Can you work these out from the model? Positions are in its coordinate system, mm. A direction names the side the tool comes from. Coordinates: 2 decimals unless noted, no trailing zeros. Loops run counter-clockwise (first coordinate to the right, second up) from the corner with the lowest first, then second, coordinate; pieces in that order, holes last. Notation, with made-up numbers: M 72.5,-25.5 L 85.5,-25.5 A15 cw 85.5,-1.5 Z; hole C 38.5,-36.75 d7. An arc over 180 degrees is marked long. Answer as a JSON object with one key per item and string values. Group by question number.
Item 1: Suppose I cut it at A-A (y = 10.5). Write out the boundary of the cut face in (x, z).
Item 2: Suppose I cut it at D-D (x = 293). Write out the boundary of the cut face in (y, z).
Item 3: We'd pull the mould along X, two halves only. Please class faces 5 (the flat face through (330.2, 2, 452)), 6 (the flat face through (0, -75, 526)), 7 (the flat face through (153, 25.4, 526)), 8 (the flat face through (279, -77, 50.8)): +X half, -X half, draft (parallel to the pull), parting line (faces both ways), or undercut.
Item 4: Suppose I cut it at B-B (z = 438). Write out the boundary of the cut face in (x, y), then the cut area to 3 significant figures.
Item 5: If I drill on line 1 (Z direction, x = 442.5, y = -31.5); line 2 (Y direction, x = 26, z = 861); line 3 (Z direction, x = 279, y = -72.5), over which ranges is the centre line in solid material (lowest first)?
Item 6: Suppose I cut it at C-C (y = -40). Write out the boundary of the cut face in (x, z), then the cut area to 3 significant figures.
Item 7: Which directions (+Z, -Z, +X, -X, +Y, -Y) give clear straight access to the entire face, cutting with the end or side of a thin tool? Please do faces 1 (the flat face through (279, 0, 592)), 2 (the flat face through (76.2, 13, 526)), 3 (the flat face through (482.6, 13, 526)), 4 (the flat face through (228.6, 9, 452)).
Item 8: I'm going to push flat-ended pins straight in: pin 1 Ø10 at (x, y) = (445, -2) entering from +Z; pin 2 Ø15 at (y, z) = (-100.5, 1103) entering from +X; pin 3 Ø20.5 at (y, z) = (15.5, 675.5) entering from -X. Where does each tip first touch, or does it pass through?
```python
from build123d import *

# Parameters (mm, degrees)
F1_DEPTH = 1066.8
F3_W     = 101.6
F3_H     = 50.8
F4_DEPTH = 152.4
F5_W     = 101.6
F5_H     = 50.8
F6_DEPTH = 177.801


with BuildPart() as f1:
    # F0 (on Top) → F1 (new body)
    with BuildSketch(Plane.XY):
        Polygon((76.2, 0), (0, 0), (0, -152.4), (558.8, -152.4), (558.8, 0), (482.6, 0), (482.6, 25.4), (330.2, 25.4), (330.2, 0), (228.6, 0), (228.6, 25.4), (76.2, 25.4), align=None)
    extrude(amount=F1_DEPTH)

    # F3 (on offset) → F4 (join)
    with BuildSketch(Plane.XZ.offset(152.4)):
        with Locations((279.4, 1092.2)):
            Rectangle(F3_W, F3_H)
    extrude(amount=-F4_DEPTH)

    # F5 (on offset) → F6 (cut, through all)
    with BuildSketch(Plane.XZ.offset(152.4)):
        with Locations((279.4, 25.4)):
            Rectangle(F5_W, F5_H)
    extrude(amount=-F6_DEPTH, mode=Mode.SUBTRACT)


solid = f1.part
```
From the geometry:
{
 "1": {"outline": "M 76.2,0 L 228.6,0 L 228.6,1066.8 L 76.2,1066.8 Z; M 330.2,0 L 482.6,0 L 482.6,1066.8 L 330.2,1066.8 Z"},
 "2": {"outline": "M -152.4,50.8 L 0,50.8 L 0,1117.6 L -152.4,1117.6 Z"},
 "3": {"face 5": "undercut", "face 6": "-X half", "face 7": "draft", "face 8": "undercut"},
 "4": {"outline": "M 0,-152.4 L 558.8,-152.4 L 558.8,0 L 482.6,0 L 482.6,25.4 L 330.2,25.4 L 330.2,0 L 228.6,0 L 228.6,25.4 L 76.2,25.4 L 76.2,0 L 0,0 Z", "area": "92,900 mm2"},
 "5": {"line 1": "0 to 1066.8", "line 2": "-152.4 to 0", "line 3": "50.8 to 1117.6"},
 "6": {"outline": "M 0,0 L 228.6,0 L 228.6,50.8 L 330.2,50.8 L 330.2,0 L 558.8,0 L 558.8,1066.8 L 330.2,1066.8 L 330.2,1117.6 L 228.6,1117.6 L 228.6,1066.8 L 0,1066.8 Z", "area": "596,000 mm2"},
 "7": {"face 1": "+Z, -Z, +Y", "face 2": "+Z, -Z, -X, +Y", "face 3": "+Z, -Z, +X, +Y", "face 4": "-Z, +Y"},
 "8": {"pin 1": "z = 1066.8", "pin 2": "x = 330.2", "pin 3": "x = 76.2"}
}
